Geometry: final body of the model. Coordinates: model frame, mm. Give positions to 0.01 mm unless a question says otherwise; leave off trailing zeros. Write each loop counter-clockwise with the first axis right and the second up, starting at its lowest first coordinate (ties: lowest second). Pieces come first, ordered by that corner, then holes. Notation, with made-up numbers: M 67.5,-9 L 102.5,-9 A28 cw 102.5,29 Z; hole C 19.5,76.25 d10. An arc over 180 degrees is marked long. Use a Markdown table: item, result. Add a question column.
(1) Cut plane A-A (z = 73.5). Output: boundary loops of the cut face in (x, y).
(2) Material intervals for L1, parallel to Z at x = 44.5, y = -1.5; L2, parallel to X at y = -1.25, z = 52.5; L3, parallel to Z at x = 52, y = -5, sorted ascending.
(3) Pin query (flat end, axial travel): pin 1 Ø1.5 at (x, y) = (62.5, -3) entering from -Z; pin 2 Ø1.5 at (x, y) = (20.5, -4.5) entering from +Z; pin 3 Ø2 at (x, y) = (17, -2.5) entering from -Z. Return the tip coordinate at first contact, or that it passes through.
(4) Cut plane B-B (y = -4). Output: boundary loops of the cut face in (x, z), plus the area to 3 significant figures.
```python
from build123d import *

# Parameters (mm, degrees)
F0_W     = 78.7
F0_H     = 156.7
F0_W_2   = 74.7
F0_H_2   = 152.7
F1_DEPTH = 6
F2_R     = 5
F3_R     = 5


with BuildPart() as f1:
    # F0 (on Front) → F1 (new body)
    with BuildSketch(Plane.XZ):
        with Locations((37.35, 76.35)):
            Rectangle(F0_W, F0_H)
        with Locations((37.35, 76.35)):
            Rectangle(F0_W_2, F0_H_2, mode=Mode.SUBTRACT)
        with Locations((37.35, 76.35)):
            Rectangle(F0_W_2, F0_H_2)
    extrude(amount=F1_DEPTH)

    # F2
    f2_edges = [f1.edges().sort_by_distance(p)[0] for p in [
        (-2, -3, -2),
        (76.7, -3, -2),
        (-2, -3, 154.7),
        (76.7, -3, 154.7),
    ]]
    fillet(f2_edges, radius=F2_R)

    # F3
    f3_edges = [f1.edges().sort_by_distance(p)[0] for p in [
        (37.35, -6, 154.7),
        (75.235534, -6, 153.235534),
        (-0.535534, -6, 153.235534),
        (76.7, -6, 76.35),
        (-2, -6, 76.35),
        (75.235534, -6, -0.535534),
        (-0.535534, -6, -0.535534),
        (37.35, -6, -2),
    ]]
    fillet(f3_edges, radius=F3_R)


solid = f1.part
```
Answer list:
| question | item | result |
|---|---|---|
| 1 | outline | M -2,-1 A5 ccw 3,-6 L 71.7,-6 A5 ccw 76.7,-1 L 76.7,0 L -2,0 Z |
| 2 | L1 | -1.97 to 154.67 |
| 2 | L2 | -1.99 to 76.69 |
| 2 | L3 | 0 to 152.7 |
| 3 | pin 1 | z = -1.84 |
| 3 | pin 2 | z = 153.88 |
| 3 | pin 3 | z = -1.97 |
| 4 | outline | M -1,3 A4 ccw 3,-1 L 71.7,-1 A4 ccw 75.7,3 L 75.7,149.7 A4 ccw 71.7,153.7 L 3,153.7 A4 ccw -1,149.7 Z |
| 4 | area | 11,900 mm² |
